Read the model definition and answer for the solid it produces. Units are mm, in the model's axes. A direction names the side the tool comes from. Coordinates: 2 decimals unless noted, no trailing zeros. Write each loop counter-clockwise with the first axis right and the second up, starting at its lowest first coordinate (ties: lowest second). Pieces come first, ordered by that corner, then holes. Notation, with made-up numbers: (57, 76) -> (115, 76) arc R13 ccw to (115, 81) -> close; hole circle Ø6 at (-17.5, 41.25). An arc over 180 degrees is marked (long way). One line per item, written item: value. Start each with the question number.
1. Find section D-D, the plane y = -1.25. Write down the section's boundary in (x, z), and give its area (3 significant figures).
2. Find section A-A, the plane z = -1.5. Write down the section's boundary in (x, y).
3. For a pull along X with two mould halves and no side action, classify faces 1 (the cylindrical face through (-1.08, -4.88, 2.46)), 2 (the flat face through (2, -2, 0)), 3 (the flat face through (0, 0, -0.8)), 4 (the cylindrical face through (-0.86, 0.27, -4.6)) as pulls with the +X half, pulls with the -X half, needs draft (parallel to the pull), parting line crosses it, or undercut.
4. For faces 5 (the flat face through (1.1, 0, -8.3)), 6 (the cylindrical face through (2.48, -0.78, -4.09)), determine the directions among +Z, -Z, +X, -X, +Y, -Y from which every point of the face is accessible in a straight line to the end or side of a thin tool.
5. Find section B-B, the plane y = 0. Write down the section's boundary in (x, z), and give its area (3 significant figures).
6. Given P1, Ø2, axis at x = 2, z = -2, coming from the +Y side; P2, Ø1.5, axis at x = 1.5, z = -1, coming from the -Y side; P3, Ø1.4, axis at x = 0, y = 0, coming from the -Z side, each flat-ended and moving along its own axis, determine where each tip first touches the part or whether it passes through.
7. Consider line 1 along Y through (x, z) = (0, -3); line 2 along Z through (x, y) = (-3.5, 2.25); line 3 along Z through (x, y) = (0, 0). Determine where each line is inside the solid, lowest interval first.
```python
from build123d import *

# Parameters (mm, degrees)
ESQUISSE1_R             = 5
BOSS_EXTRU_1_DEPTH      = 5
ESQUISSE2_R             = 2.6
BOSS_EXTRU_2_DEPTH      = 8.3
ESQUISSE3_R             = 0.9
ENL_V_MAT_EXTRU_1_DEPTH = 7.5


with BuildPart() as part:
    # Esquisse1 → Boss.-Extru.1 (new body)
    with BuildSketch(Plane.XY):
        Circle(ESQUISSE1_R)
    extrude(amount=BOSS_EXTRU_1_DEPTH)

    # Esquisse2 → Boss.-Extru.2 (add)
    with BuildSketch(Plane(origin=(0, 0, 0), x_dir=(-1, 0, 0), z_dir=(0, 0, -1))):
        with Locations(Location((0, 0, 0), (0, 0, 180))):
            Circle(ESQUISSE2_R)
    extrude(amount=BOSS_EXTRU_2_DEPTH)

    # Esquisse3 → Enlèv. mat.-Extru.1 (cut)
    with BuildSketch(Plane(origin=(0, 0, -8.3), x_dir=(-1, 0, 0), z_dir=(0, 0, -1))):
        Circle(ESQUISSE3_R)
    extrude(amount=-ENL_V_MAT_EXTRU_1_DEPTH, mode=Mode.SUBTRACT)


solid = part.part
```
Answer block:
1. outline: (-4.84, 0) -> (-2.28, 0) -> (-2.28, -8.3) -> (2.28, -8.3) -> (2.28, 0) -> (4.84, 0) -> (4.84, 5) -> (-4.84, 5) -> close
1. area: 86.3 mm2
2. outline: circle Ø5.2 at (0, 0); hole circle Ø1.8 at (0, 0)
3. face 1: parting line crosses it
3. face 2: needs draft
3. face 3: undercut
3. face 4: undercut
4. face 5: -Z, +X, -X, +Y, -Y
4. face 6: -Z
5. outline: (-5, 0) -> (-2.6, 0) -> (-2.6, -8.3) -> (-0.9, -8.3) -> (-0.9, -0.8) -> (0.9, -0.8) -> (0.9, -8.3) -> (2.6, -8.3) -> (2.6, 0) -> (5, 0) -> (5, 5) -> (-5, 5) -> close
5. area: 79.7 mm2
6. P1: stops at y = 2.4
6. P2: stops at y = -2.49
6. P3: stops at z = -0.8
7. line 1: y = -2.6 to -0.9, 0.9 to 2.6
7. line 2: z = 0 to 5
7. line 3: z = -0.8 to 5
